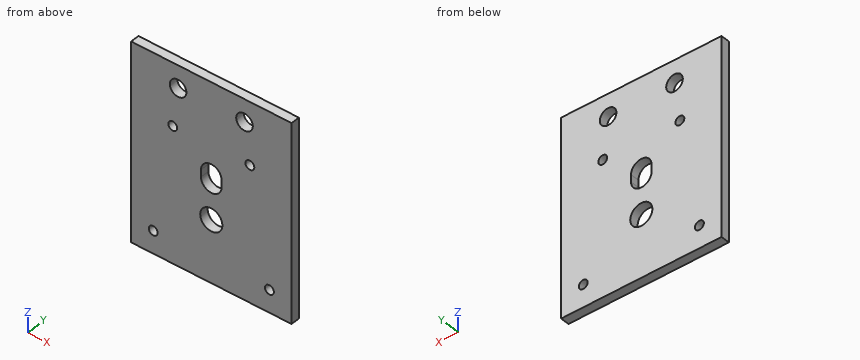
```python
from build123d import *

# Parameters (mm, degrees)
BOSS_EXTRUDE1_DEPTH          = 5.08
F_3_8_0_375_DIAMETER_HOLE1_D = 9.525
F_3_8_0_375_DIAMETER_HOLE2_D = 9.525
SKETCH8_R                    = 6.35
CUT_EXTRUDE1_DEPTH           = 1371.578062618
SKETCH9_R                    = 2.5527
CUT_EXTRUDE2_DEPTH           = 1371.578062618
SKETCH10_OUTSIDE_W           = 496.242
SKETCH10_OUTSIDE_H           = 717.956
SKETCH10_OUTSIDE_W_2         = 92.023830603
SKETCH10_OUTSIDE_H_2         = 111.269815094
CUT_EXTRUDE3_DEPTH           = 1371.578062618


with BuildPart() as part:
    # Sketch1 → Boss-Extrude1 (new body)
    with BuildSketch(Plane(origin=(0, 0, 0), x_dir=(1, 0, 0), z_dir=(0, 1, 0))):
        with BuildLine():
            Line((186.706216966, -778.102360844), (-171.269771153, -778.102360844))
            add(Edge.make_bspline(
                [(-171.269771153, -778.102360844), (-159.707774454, -836.134775395), (-146.81892484, -893.9188082), (-132.611103769, -951.360767835), (-118.403260068, -1008.802818957), (-102.873342202, -1065.933903144), (-86.045569786, -1122.663773012), (-74.990089761, -1159.934062127), (-63.371281317, -1197.041907081), (-51.194215445, -1233.960969312), (-45.100567198, -1252.436009294), (-38.866841431, -1270.865430421), (-32.494599583, -1289.246240662), (-26.120797202, -1307.631552278), (-20.652525047, -1326.386680917), (-12.917829919, -1344.242199148)],
                knots=[0, 0, 0, 0, 0.177518923, 0.177518923, 0.177518923, 0.355038121, 0.355038121, 0.355038121, 0.471646972, 0.471646972, 0.471646972, 0.529995372, 0.529995372, 0.529995372, 0.588358391, 0.588358391, 0.588358391, 0.588358391], degree=3))
            ThreePointArc((-12.917829919, -1344.242199148), (7.718222897, -1357.79203399), (28.354275723, -1344.242199164))
            add(Edge.make_bspline(
                [(28.354275723, -1344.242199164), (38.120725658, -1321.696381858), (44.939237661, -1298.079369173), (60.823654171, -1251.671639351), (68.544496879, -1228.393431097), (91.029194373, -1158.368706478), (105.122355407, -1111.420274649), (144.723795491, -969.782644477), (167.537266257, -874.315888923), (186.706216966, -778.102360844)],
                knots=[0, 0, 0, 0, 0.125, 0.125, 0.25, 0.25, 0.5, 0.5, 1, 1, 1, 1], degree=3))
        make_face()
    extrude(amount=BOSS_EXTRUDE1_DEPTH)

    # 3_8 _0.375_ Diameter Hole1 (through all)
    with Locations(Plane(origin=(0, 5.08, 0), x_dir=(1, 0, 0), z_dir=(0, 1, 0))):
        with Locations((7.718222897, -1326.04203399), (7.718222897, -1300.64203399)):
            Hole(F_3_8_0_375_DIAMETER_HOLE1_D / 2)

    # 3_8 _0.375_ Diameter Hole2 (through all)
    with Locations(Plane(origin=(0, 5.08, 0), x_dir=(1, 0, 0), z_dir=(0, 1, 0))):
        with Locations((-49.431777094, -970.44203399), (-49.431777094, -1008.54203399), (64.868222906, -970.44203399), (64.868222906, -1008.54203399), (-11.331777094, -1205.39203399), (26.768222906, -1205.39203399)):
            Hole(F_3_8_0_375_DIAMETER_HOLE2_D / 2)

    # Sketch8 → Cut-Extrude1 (cut, through all)
    with BuildSketch(Plane(origin=(0, 5.08, 0), x_dir=(1, 0, 0), z_dir=(0, 1, 0))):
        with Locations(Location((7.718222906, -1141.89203399, 0), (0, 0, 270))):
            Circle(SKETCH8_R)
        with BuildLine():
            Line((1.812722906, -1166.764753462), (1.812722906, -1162.739314519))
            ThreePointArc((1.812722906, -1162.739314519), (7.718222906, -1156.833814519), (13.623722906, -1162.739314519))
            Line((13.623722906, -1162.739314519), (13.623722906, -1166.764753462))
            ThreePointArc((13.623722906, -1166.764753462), (7.718222906, -1172.670253462), (1.812722906, -1166.764753462))
        make_face()
    extrude(amount=-CUT_EXTRUDE1_DEPTH, mode=Mode.SUBTRACT)

    # Sketch9 → Cut-Extrude2 (cut, through all)
    with BuildSketch(Plane(origin=(0, 5.08, 0), x_dir=(1, 0, 0), z_dir=(0, 1, 0))):
        with Locations(Location((-14.396929121, -1183.022218896, 0), (0, 0, 270))):
            Circle(SKETCH9_R)
        with Locations(Location((29.833374932, -1183.022218896, 0), (0, 0, 270))):
            Circle(SKETCH9_R)
        with Locations(Location((41.030138207, -1119.522218896, 0), (0, 0, 270))):
            Circle(SKETCH9_R)
        with Locations(Location((-25.593692396, -1119.522218896, 0), (0, 0, 270))):
            Circle(SKETCH9_R)
    extrude(amount=-CUT_EXTRUDE2_DEPTH, mode=Mode.SUBTRACT)

    # Sketch10 outside → Cut-Extrude3 (cut, through all)
    with BuildSketch(Plane(origin=(0, 5.08, 0), x_dir=(1, 0, 0), z_dir=(0, 1, 0))):
        with Locations((7.718, -1067.947)):
            Rectangle(SKETCH10_OUTSIDE_W, SKETCH10_OUTSIDE_H)
        with Locations((7.718222905, -1162.457126443)):
            Rectangle(SKETCH10_OUTSIDE_W_2, SKETCH10_OUTSIDE_H_2, mode=Mode.SUBTRACT)
    extrude(amount=-CUT_EXTRUDE3_DEPTH, mode=Mode.SUBTRACT)


solid = part.part
```
Work out the finished part from the listing and answer in its coordinate system (mm). Give positions to 0.01 mm unless a question says otherwise; leave off trailing zeros. Loops run counter-clockwise (first coordinate to the right, second up) from the corner with the lowest first, then second, coordinate; pieces in that order, holes last. Notation, with made-up numbers: (78, 73) -> (134, 73) arc R16 ccw to (134, 84) -> close; hole circle Ø4 at (29, 37.25). An arc over 180 degrees is marked (long way). Write item = value, one per line. Start each with the question number.
(1) Find section B-B on y = 3.7. Give the number of separate pieces and of enclosed holes in the cut face, and give its area (3 significant figures).
(2) Find the intervals of material crossed by probe 1 along Z at (x, y) = (-11.5, 1.2); probe 2 along Z at (x, y) = (29.5, 4.75); probe 3 along X at (y, z) = (3.85, 1167), in increasing order. Write a range as from..to.
(3) Find section A-A on z = 1143.5. Give the vertices of the cut face in (x, y), and give its area (3 significant figures).
(4) Find section C-C on x = 24.5. Give the vertices of the cut face in (y, z).
From the geometry:
q1.separate_pieces = 1
q1.enclosed_holes = 8
q1.area = 9,730 mm^2
q2.probe_1 = 1106.82..1200.63, 1210.15..1218.09
q2.probe_2 = 1106.82..1180.49, 1185.55..1201.49, 1209.29..1218.09
q2.probe_3 = -38.29..1.82, 13.62..53.73
q3.outline = (-38.29, 0) -> (1.58, 0) -> (1.58, 5.08) -> (-38.29, 5.08) -> close; (13.86, 0) -> (53.73, 0) -> (53.73, 5.08) -> (13.86, 5.08) -> close
q3.area = 405 mm^2
q4.outline = (0, 1106.82) -> (5.08, 1106.82) -> (5.08, 1201.2) -> (0, 1201.2) -> close; (0, 1209.58) -> (5.08, 1209.58) -> (5.08, 1218.09) -> (0, 1218.09) -> close
